```python
from build123d import *

# Parameters (mm, degrees)
F0_R     = 11.0000034
F1_DEPTH = 6.35
F2_SIZE  = 3.17499


# Not quite as in the source:
# - a fillet or chamfer is up to 0.001 mm smaller than in the source, because OpenCascade refuses the exact size


with BuildPart() as f1:
    # F0 (on Top) → F1 (new body)
    with BuildSketch(Plane.XY):
        with BuildLine():
            Line((-1.1111190304, 28.591448421), (-5.08, 14.3684097937))
            ThreePointArc((-5.08, 14.3684097937), (-8.9578472449, 12.3294189943), (-12.0953634317, 9.2714499112))
            Line((-12.0953634317, 9.2714499112), (-26.8487286679, 9.8919804501))
            Line((-26.8487286679, 9.8919804501), (-29.9476720311, 13.9172692636))
            Line((-29.9476720311, 13.9172692636), (-41.2574764774, 13.4053667244))
            Line((-41.2574764774, 13.4053667244), (-32.4085412404, 6.3434926108))
            Line((-32.4085412404, 6.3434926108), (-27.5354379943, 7.7785064617))
            Line((-27.5354379943, 7.7785064617), (-15.2349760945, -0.3912842944))
            ThreePointArc((-15.2349760945, -0.3912842944), (-14.4941013083, -4.7094189943), (-12.5553457071, -8.6383386236))
            Line((-12.5553457071, -8.6383386236), (-17.7045459019, -22.4778682868))
            Line((-17.7045459019, -22.4778682868), (-22.4904492218, -24.1812559153))
            Line((-22.4904492218, -24.1812559153), (-25.4985227531, -35.0957057161))
            Line((-25.4985227531, -35.0957057161), (-16.0478099898, -28.8621073099))
            Line((-16.0478099898, -28.8621073099), (-15.9067175452, -23.784067046))
            Line((-15.9067175452, -23.784067046), (-4.3357330442, -14.6102367869))
            ThreePointArc((-4.3357330442, -14.6102367869), (0, -15.24), (4.3357330442, -14.6102367869))
            Line((4.3357330442, -14.6102367869), (15.9067175452, -23.784067046))
            Line((15.9067175452, -23.784067046), (16.0478099898, -28.8621073099))
            Line((16.0478099898, -28.8621073099), (25.4985227531, -35.0957057161))
            Line((25.4985227531, -35.0957057161), (22.4904492218, -24.1812559153))
            Line((22.4904492218, -24.1812559153), (17.7045459019, -22.4778682868))
            Line((17.7045459019, -22.4778682868), (12.5553457071, -8.6383386236))
            ThreePointArc((12.5553457071, -8.6383386236), (14.4941013083, -4.7094189943), (15.2349760945, -0.3912842944))
            Line((15.2349760945, -0.3912842944), (27.5354379943, 7.7785064617))
            Line((27.5354379943, 7.7785064617), (32.4085412404, 6.3434926108))
            Line((32.4085412404, 6.3434926108), (41.2574764774, 13.4053667244))
            Line((41.2574764774, 13.4053667244), (29.9476720311, 13.9172692636))
            Line((29.9476720311, 13.9172692636), (26.8487286679, 9.8919804501))
            Line((26.8487286679, 9.8919804501), (12.0953634317, 9.2714499112))
            ThreePointArc((12.0953634317, 9.2714499112), (8.9578472449, 12.3294189943), (5.08, 14.3684097937))
            Line((5.08, 14.3684097937), (1.1111190304, 28.591448421))
            Line((1.1111190304, 28.591448421), (3.9817700226, 32.7826013508))
            Line((3.9817700226, 32.7826013508), (0, 43.3806779834))
            Line((0, 43.3806779834), (-3.9817700226, 32.7826013508))
            Line((-3.9817700226, 32.7826013508), (-1.1111190304, 28.591448421))
        make_face()
        Circle(F0_R, mode=Mode.SUBTRACT)
    extrude(amount=F1_DEPTH)

    # F2 (size 3.175 in the source; OpenCascade refuses exactly that, so slightly less here)
    f2_edges = [f1.edges().sort_by_distance(p)[0] for p in [
        (35.602574, 13.661318, 6.35),
        (35.602574, 13.661318, 0),
        (36.833009, 9.87443, 6.35),
        (36.833009, 9.87443, 0),
        (1.990885, 38.08164, 6.35),
        (1.990885, 38.08164, 0),
        (23.994486, -29.638481, 6.35),
        (23.994486, -29.638481, 0),
        (-35.602574, 13.661318, 6.35),
        (-35.602574, 13.661318, 0),
        (-1.990885, 38.08164, 6.35),
        (-1.990885, 38.08164, 0),
        (-23.994486, -29.638481, 6.35),
        (-23.994486, -29.638481, 0),
        (-36.833009, 9.87443, 6.35),
        (-36.833009, 9.87443, 0),
        (-20.773166, -31.978907, 6.35),
        (-20.773166, -31.978907, 0),
        (20.773166, -31.978907, 6.35),
        (20.773166, -31.978907, 0),
    ]]
    chamfer(f2_edges, length=F2_SIZE)


solid = f1.part
```
Here's how the part is built. I have some questions about the finished solid (model axes, mm). A direction names the side the tool comes from. Give positions to 0.01 mm unless a question says otherwise; leave off trailing zeros. Order: outer loops, then holes, each group sorted by start corner. A loop starts at its lowest first (then second) coordinate and runs counter-clockwise, first axis right, second up. Notation, with made-up numbers: (7.5, 29.5) - (43.5, 29.5) arc R23 cw to (43.5, 56.5) - close; hole circle Ø3 at (-33, -5). An arc over 180 degrees is marked (long way). Answer as a JSON object with one key per item and string values. Group by question number.
Item 1: If we mould it in two halves opening along X, with no side actions, what happens to faces 6 (the flat face through (-1.7, 35.28, 1.92)), 7 (the flat face through (-28.032, 11.429, 3.131)), 8 (the flat face through (33.93, 9.166, 4.432)), 9 (the flat face through (10, -19.1, 3.1))? For each: pulls with the +X half, pulls with the -X half, needs draft (parallel to the pull), parting line crosses it, or undercut.
Item 2: For P1, Ø1.5, axis at y = 9.5, z = 1.5, coming from the +X side; P2, Ø1.5, axis at x = -12.5, y = -22.5, coming from the +Z side, each with a flat end and sliding along its axis, tell me the tip position at first contact or that it passes through.
Item 3: If we section it at B-B on x = 13.5: Please give me the cut outline in (y, z), and give its area (3 significant figures).
Item 4: Which directions (+Z, -Z, +X, -X, +Y, -Y) give clear straight access to the entire face, cutting with the end or side of a thin tool? Please do faces 1 (the flat face through (-22.062, -27.359, 1.918)), 2 (the flat face through (22.113, -27.541, 1.918)), 3 (the flat face through (19.2, -29.44, 4.43)), 4 (the flat face through (-29.5, 7.2, 3.1)), 5 (the cylindrical face through (14.475, -4.768, 3.131)).
Item 5: If we section it at A-A on y = -20.5: Please give me the cut outline in (x, z), and give its area (3 significant figures).
Item 6: Please list where these lines run through material, in increasing order: probe 1 along X at (y, z) = (-8, 6); probe 2 along X at (y, z) = (-25, 3); probe 3 along Y at (x, z) = (-26, 5.5).
Result set:
{
 "1": {"face 6": "pulls with the -X half", "face 7": "undercut", "face 8": "pulls with the +X half", "face 9": "undercut"},
 "2": {"P1": "x = 35.2", "P2": "through"},
 "3": {"outline": "(-21.88, 0) - (-11.18, 0) - (-11.18, 6.35) - (-21.88, 6.35) - close; (-7.07, 0) - (9.33, 0) - (9.33, 6.35) - (-7.07, 6.35) - close", "area": "172 mm²"},
 "4": {"face 1": "-Z, -X", "face 2": "-Z, +X", "face 3": "+Z, -Y", "face 4": "+Z, -Z, -Y", "face 5": "+Z, -Z, +X"},
 "5": {"outline": "(-16.97, 0) - (-11.76, 0) - (-11.76, 6.35) - (-16.97, 6.35) - close; (11.76, 0) - (16.97, 0) - (16.97, 6.35) - (11.76, 6.35) - close", "area": "66.1 mm²"},
 "6": {"probe 1": "-12.97 to -7.55, 7.55 to 12.97", "probe 2": "-22.53 to -15.94, 15.94 to 22.53", "probe 3": "6.76 to 9.86"}
}
